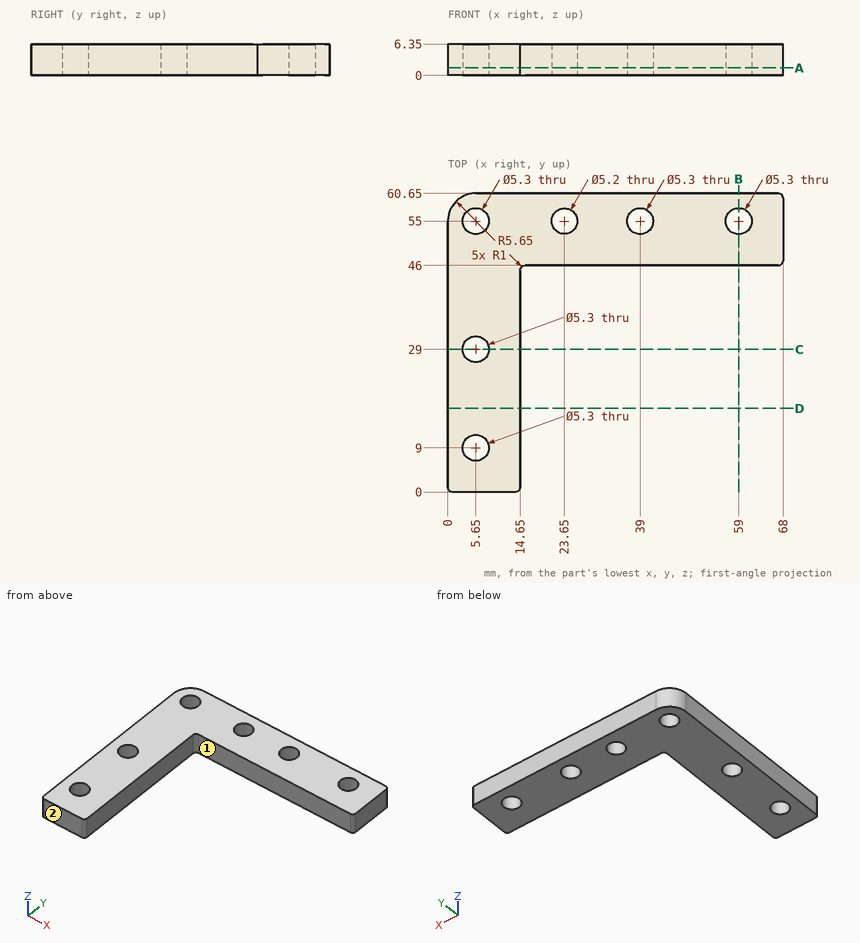
Design review of the part shown in the three views and the two pictorial views. Dimensions are in mm from the part's minimum x, y and z. A direction names the side the tool comes from. Coordinates: 2 decimals unless noted, no trailing zeros. Order: outer loops, then holes, each group sorted by start corner. A loop starts at its lowest first (then second) coordinate and runs counter-clockwise, first axis right, second up.
1) Clearance check with flat-ended pins moving along their axes: pin 1 (2 mm diameter, centred on y = 22.5, z = 5, fed in from +X); pin 2 (1 mm diameter, centred on x = 47, z = 3, fed in from -Y). State where each tip first meets the part, or that it passes through.
2) Wall thickness on line 1 along Y through (x, z) = (5.5, 5.25); line 2 along X through (y, z) = (29, 3.5); line 3 along Y through (x, z) = (59, 4.75): over which ranges is each line inside the solid? List them lowest first.
3) For the marked faces 1 and 2, list the 3-axis set-ups (+Z, -Z, +X, -X, +Y, -Y) from which the entire face can be reached by the end or side of a thin tool; tool diameter is ignored.
4) Take a section at A-A, the plane z = 1.5. Give the boundary of the cut face in (x, y).
5) Take a section at D-D, the plane y = 17. Give the boundary of the cut face in (x, z).
6) Take a section at C-C, the plane y = 29. Give the boundary of the cut face in (x, z).
7) Take a section at B-B, the plane x = 59. Give the boundary of the cut face in (y, z).
Returned:
1. pin 1: stops at x = 14.65
1. pin 2: stops at y = 46
2. line 1: y = 0 to 6.35, 11.65 to 26.35, 31.65 to 52.35, 57.65 to 60.65
2. line 2: x = 0 to 3, 8.3 to 14.65
2. line 3: y = 46 to 52.35, 57.65 to 60.65
3. face 1: +Z, -Z, +X, -Y
3. face 2: +Z, -Z, +X, -X, -Y
4. outline: (0, 1) arc R1 ccw to (1, 0) - (13.65, 0) arc R1 ccw to (14.65, 1) - (14.65, 45) arc R1 cw to (15.65, 46) - (67, 46) arc R1 ccw to (68, 47) - (68, 59.65) arc R1 ccw to (67, 60.65) - (5.65, 60.65) arc R5.65 ccw to (0, 55) - close; hole circle Ø5.3 at (5.65, 9); hole circle Ø5.3 at (5.65, 29); hole circle Ø5.3 at (5.65, 55); hole circle Ø5.2 at (23.65, 55); hole circle Ø5.3 at (39, 55); hole circle Ø5.3 at (59, 55)
5. outline: (0, 0) - (14.65, 0) - (14.65, 6.35) - (0, 6.35) - close
6. outline: (0, 0) - (3, 0) - (3, 6.35) - (0, 6.35) - close; (8.3, 0) - (14.65, 0) - (14.65, 6.35) - (8.3, 6.35) - close
7. outline: (46, 0) - (52.35, 0) - (52.35, 6.35) - (46, 6.35) - close; (57.65, 0) - (60.65, 0) - (60.65, 6.35) - (57.65, 6.35) - close
